Part model, mm, in its own coordinate system. Face numbers are marked on the shaded views. A direction names the side the tool comes from. Give positions to 0.01 mm unless a question says otherwise; leave off trailing zeros. Order: outer loops, then holes, each group sorted by start corner. A loop starts at its lowest first (then second) coordinate and runs counter-clockwise, first axis right, second up.
1. Drop flat-ended pins along their axis: pin 1 Ø0.5 at (y, z) = (3.5, 0) entering from -X; pin 2 Ø4 at (x, y) = (-0.5, 4) entering from +Z; pin 3 Ø2.5 at (x, y) = (0, 3.5) entering from -Z. Give the stop position or say it passes through.
2. Slice it at A-A on z = 0. List the corners of the cut face in (x, y), and give its area (3 significant figures).
3. Mould opens along X. For the marked faces 3, 4 and 5 say: +X half, -X half, draft (parallel to the pull), parting line (faces both ways), or undercut.
4. Probe line 1 (Z direction, x = 0, y = 9.5); line 2 (Z direction, x = -2, y = 1); line 3 (X direction, y = 8.5, z = -9.5). List the from-to ranges inside material, lowest first.
5. Which spindle directions (+Z, -Z, +X, -X, +Y, -Y) get a long thin tool onto all of the face, cutting with end or side? Do the marked faces 1 and 2. Say none if no direction does.
Autodesk Inventor part; units mm, degrees
ref_plane "Work Plane1" through (5.75, 10, 8.5) normal (0, -1, 0) x (1, 0, 0)
ref_plane "YZ Plane" through (0, 0, 0) normal (1, 0, 0) x (0, 1, 0)
ref_plane "XZ Plane" through (0, 0, 0) normal (0, 1, 0) x (-1, 0, 0)
sketch "Sketch2" plane through (0, 0, 0) normal (1, 0, 0) x (0, 1, 0)
  point P0 (0, 0)
sketch "Sketch3" plane through (0, 0, 0) normal (1, 0, 0) x (0, 1, 0)
  arc A0 (10, 8.5) -> (10, -8.5) centre (25.8666, 0) ccw
  arc A1 (10, 8.5) -> (0, 11.7145) centre (1, -2.3365) ccw
  line L0 (0, 11.7145) -> (0, -11.7145)
  line L1 (0, 0) -> (7.8666, 0)
  line L2 (2.6813, 11.75) -> (0, 11.75) construction
  arc A2 (0, -11.7145) -> (10, -8.5) centre (1, 2.3365) ccw
  line L3 (2.6813, -11.75) -> (0, -11.75) construction
  dimension "d1" = 10
  dimension "d2" = 23.5
  dimension "d3" = 1
  dimension "d4" = 17
  dimension "d5" = 18
extrude "Extrusion1" add sketch "Sketch3" along normal mid plane 11.5
sketch "Sketch4" plane through (-5.75, 0, -11.7145) normal (0, -1, 0) x (1, 0, 0)
  line L0 (4.75, 13.7145) -> (6.75, 13.7145)
  line L1 (6.75, 13.7145) -> (6.75, 9.7145)
  line L2 (6.75, 9.7145) -> (4.75, 9.7145)
  line L3 (4.75, 9.7145) -> (4.75, 13.7145)
  line L4 (4.75, 13.7145) -> (6.75, 9.7145) construction
  line L5 (6.75, 13.7145) -> (4.75, 9.7145) construction
  point P0 (5.75, 11.7145)
  dimension "d8" = 2
  dimension "d9" = 4
extrude "Extrusion2" cut sketch "Sketch4" against normal blind 6
sketch "Sketch5" plane through (5.75, 0, 0) normal (1, 0, 0) x (0, 0, -1)
  line L0 (11.7145, 0) -> (-11.7145, 0)
  line L1 (-0.5, 0) -> (0.5, 0)
  line L2 (0.5, 0) -> (0.5, 9.525)
  line L3 (0.5, 9.525) -> (-0.5, 9.525)
  line L4 (-0.5, 9.525) -> (-0.5, 0)
  point P0 (0, 0)
  point P1 (0, 0)
  dimension "d12" = 1
extrude "Extrusion3" cut sketch "Sketch5" against normal blind 0.1
mirror "Mirror1" about plane through (0, 0, 0) normal (1, 0, 0) of "Extrusion3"
ref_plane "Work Plane1" through (5.75, 10, 8.5) normal (0, -1, 0) x (1, 0, 0)
sketch "Sketch6" plane through (5.75, 10, 8.5) normal (0, -1, 0) x (1, 0, 0)
  line L0 (-11.4, -8) -> (-11.4, -9)
  line L1 (-11.4, -8) -> (-0.1, -8)
  line L2 (-0.1, -8) -> (-0.1, -9)
  line L3 (-0.1, -9) -> (-11.4, -9)
  line L4 (-11.4, -9) -> (-11.4, -8)
  point P0 (-5.75, -8.5)
extrude "Extrusion4" cut sketch "Sketch6" along normal blind 2.2
fillet "Fillet1" radius 0.1 10 edges at (-5.75, 5.3108, -11.0742) (5.75, 5.3108, -11.0742) (0, 10, -8.5) (5.75, 8.4707, -4.6239) (-5.75, 8.4707, -4.6239) (-5.75, 8.4707, 4.6239) (5.75, 8.4707, 4.6239) (-5.75, 5.3108, 11.0742) (0, 10, 8.5) (5.75, 5.3108, 11.0742)
properties part number "Cup"
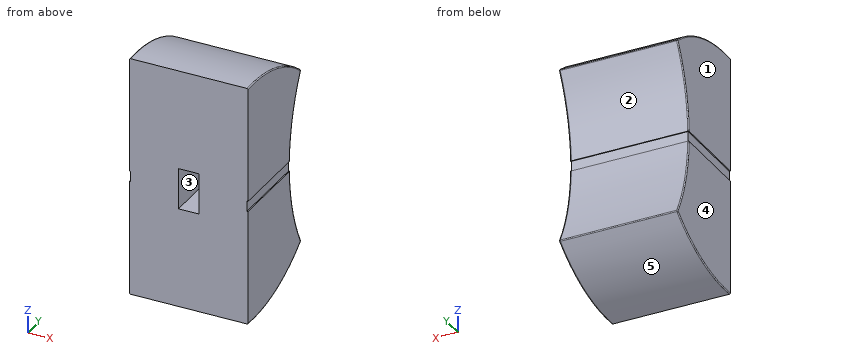
Data:
1. pin 1: stops at x = -5.65
1. pin 2: stops at z = 11.71
1. pin 3: stops at z = -11.69
2. outline: (-5.65, 0) - (-1, 0) - (-1, 6) - (1, 6) - (1, 0) - (5.65, 0) - (5.65, 7.8) - (-5.65, 7.8) - close
2. area: 76.1 mm2
3. face 3: undercut
3. face 4: -X half
3. face 5: draft
4. line 1: z = -8.9 to -7.49, 7.49 to 8.9
4. line 2: z = -11.75 to 11.75
4. line 3: x = -5.75 to 5.75
5. face 1: +Z, -Z, -X, +Y, -Y
5. face 2: +X, -X, +Y
